Input: part model. Units: mm. Frame: model coordinates. Face numbers are marked on the shaded views. A direction names the side the tool comes from. Give positions to 0.01 mm unless a question says otherwise; leave off trailing zeros. Loops run counter-clockwise (first coordinate to the right, second up) from the corner with the lowest first, then second, coordinate; pieces in that order, holes last. Notation, with made-up numbers: M 37.5,-5.75 L 76.5,-5.75 A33 ccw 76.5,29.25 Z; hole C 9,64.5 d5. An arc over 180 degrees is marked long. Answer as a JSON object with one key per item and string values. Group by question number.
1) Section query A-A on x = 0. Return loops of the section in (y, z), plus the area to 4 significant figures.
2) Section query C-C on z = -20.5. Return loops of the section in (x, y), plus the area to 3 significant figures.
3) Section query B-B on z = 20.5. Return loops of the section in (x, y) (3 decimals), plus the area to 3 significant figures.
4) Ray query, L1, parallel to Y at x = 8, z = -20.5; L2, parallel to Z at x = -9, y = -23.25; L3, parallel to X at y = -26.5, z = 17. Return the intervals inside material, ascending.
5) Draft query along Y for the marked faces 1, 2, 3 and 4. Return one class per face: +Y half, -Y half, draft (parallel to the pull), parting line (faces both ways), or undercut.
6) First-contact query: P1, Ø1, axis at x = -10.5, y = -5, coming from the -Z side; P2, Ø1.5, axis at x = 0, z = -20.5, coming from the -Y side; P3, Ø3, axis at x = -4, y = -17, coming from the -Z side; P4, Ø2, axis at x = -1, y = -28, coming from the -Z side. Flat tips, straight axial feed; report the tip coordinate or a pass-through.
7) Access query for the marked faces 5, 6, 7, 8 and 9. Directions: +Z, -Z, +X, -X, +Y, -Y. A direction counts if a zero-diameter tool reaches every point of the face in a straight line with its end or side. Return the directions, or none.
8) Section query D-D on x = -8. Return loops of the section in (y, z).
from build123d import *

# Parameters (mm, degrees)
F1_DEPTH = 10
F2_D     = 2.5
F3_W     = 20
F3_H     = 10
F4_DEPTH = 20
F6_DEPTH = 20
F7_R     = 5


with BuildPart() as f1:
    # F0 (on Front) → F1 (new body)
    with BuildSketch(Plane.XZ):
        with BuildLine():
            Line((-10, 34), (-10, 24))
            ThreePointArc((-10, 24), (0, -26), (10, 24))
            Line((10, 24), (10, 34))
            Line((10, 34), (-10, 34))
        make_face()
    extrude(amount=F1_DEPTH)

    # F2 (through all)
    with Locations(Plane(origin=(0, 0, 0), x_dir=(1, 0, 0), z_dir=(0, 1, 0))):
        with Locations((0, -20.5), (0, 20.5)):
            Hole(F2_D / 2)

    # F3 (on face) → F4 (join)
    with BuildSketch(Plane.XZ.offset(10)):
        with Locations((0, 29)):
            Rectangle(F3_W, F3_H)
    extrude(amount=F4_DEPTH)

    # F5 (on face) → F6 (join, through all)
    with BuildSketch(Plane(origin=(-10, 0, 0), x_dir=(0, -1, 0), z_dir=(-1, 0, 0))):
        Polygon((30, 14), (30, 24), (24, 24), (23.5, 14), align=None)
    extrude(amount=-F6_DEPTH)

    # F7
    f7_edges = [f1.edges().sort_by_distance(p)[0] for p in [
        (10, -5, 24),
        (-10, -5, 24),
    ]]
    fillet(f7_edges, radius=F7_R)


solid = f1.part
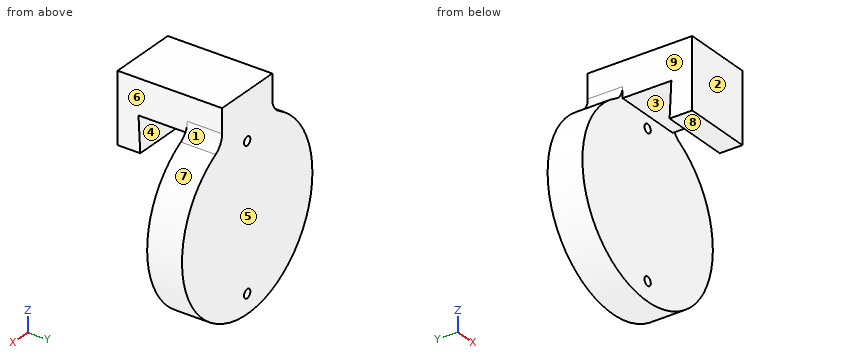
Output:
{
 "1": {"outline": "M -30,14 L -23.5,14 L -24,24 L -10,24 L -10,21.75 L 0,21.75 L 0,34 L -30,34 Z; M -10,-26 L 0,-26 L 0,-21.75 L -10,-21.75 Z; M -10,-19.25 L 0,-19.25 L 0,19.25 L -10,19.25 Z", "area": "812.5 mm^2"},
 "2": {"outline": "M -15.99,-10 L -1.25,-10 L -1.25,0 L -15.99,0 Z; M 1.25,-10 L 15.99,-10 L 15.99,0 L 1.25,0 Z", "area": "295 mm^2"},
 "3": {"outline": "M -15.992,-10 L -1.25,-10 L -1.25,0 L -15.992,0 Z; M -10,-30 L 10,-30 L 10,-23.825 L -10,-23.825 Z; M 1.25,-10 L 15.992,-10 L 15.992,0 L 1.25,0 Z", "area": "418 mm^2"},
 "4": {"L1": "y = -10 to 0", "L2": "z = 24 to 34", "L3": "x = -10 to 10"},
 "5": {"face 1": "draft", "face 2": "-Y half", "face 3": "undercut", "face 4": "undercut"},
 "6": {"P1": "stops at z = -24", "P2": "passes through", "P3": "stops at z = 24", "P4": "stops at z = 14"},
 "7": {"face 5": "+Z, -Z, +X, -X, +Y", "face 6": "+Z, +X, -Y", "face 7": "+Y, -Y", "face 8": "-Z, +X, -X, -Y", "face 9": "+Z, -X, -Y"},
 "8": {"outline": "M -30,14 L -23.5,14 L -24,24 L -10,24 L -10,-24.74 L 0,-24.74 L 0,34 L -30,34 Z"}
}
